from build123d import *

# Parameters (mm, degrees)
F0_R     = 21.614199
F1_DEPTH = 25.4


with BuildPart() as f1:
    # F0 (on Front) → F1 (new body)
    with BuildSketch(Plane.XZ):
        Polygon((-35.520531, 23.765538), (-35.520531, 0), (-35.520531, -26.832053), (-10.988366, -44.209), (-10.988366, -75.385295), (13.543796, -75.385295), (13.543796, -44.209), (38.075965, -26.832053), (38.075965, 0), (38.075965, 23.765538), align=None)
        Circle(F0_R, mode=Mode.SUBTRACT)
    extrude(amount=F1_DEPTH)


solid = f1.part
Here's how the part is built. I have some questions about the finished solid (model axes, mm). A direction names the side the tool comes from. Coordinates: 2 decimals unless noted, no trailing zeros. Order: outer loops, then holes, each group sorted by start corner. A loop starts at its lowest first (then second) coordinate and runs counter-clockwise, first axis right, second up.
Item 1: If we section it at A-A on y = -7.5: List the corners of the cut face in (x, z) for me.
Result sheet:
outline: (-35.52, -26.83) - (-10.99, -44.21) - (-10.99, -75.39) - (13.54, -75.39) - (13.54, -44.21) - (38.08, -26.83) - (38.08, 23.77) - (-35.52, 23.77) - close; hole circle Ø43.23 at (0, 0)
Item 2: I need wall thicknesses on line 1 (Z direction, x = 0, y = -13); line 2 (X direction, y = -22, z = -1); line 3 (X direction, y = -8.5, z = -56). Which ranges of each line are inside material? Lowest first, please.
Result sheet:
line 1: z = -75.39 to -21.61, 21.61 to 23.77
line 2: x = -35.52 to -21.59, 21.59 to 38.08
line 3: x = -10.99 to 13.54
Item 3: For faces 1 (the face through (13.544, -13, -60)), 2 (the face through (1, -13, -75.385)), which set-ups out of +Z, -Z, +X, -X, +Y, -Y let a thin tool reach every point of the face, with its end or its side?
Result sheet:
face 1: -Z, +X, +Y, -Y
face 2: -Z, +X, -X, +Y, -Y
Item 4: If we section it at D-D on x = 30.5: List the corners of the cut face in (y, z) for me.
Result sheet:
outline: (-25.4, -32.2) - (0, -32.2) - (0, 23.77) - (-25.4, 23.77) - close
Item 5: For P1, Ø2, axis at x = -14, y = -20.5, coming from the -Z side; P2, Ø1, axis at y = -6, z = -31.5, coming from the +X side; P3, Ø5, axis at x = -19.5, y = -5.5, coming from the -Z side, each with a flat end and sliding along its axis, tell me the tip position at first contact or that it passes through.
Result sheet:
P1: stops at z = -42.78
P2: stops at x = 32.19
P3: stops at z = -39.95
Item 6: If we section it at C-C on x = 0: List the corners of the cut face in (y, z) for me.
Result sheet:
outline: (-25.4, -75.39) - (0, -75.39) - (0, -21.61) - (-25.4, -21.61) - close; (-25.4, 21.61) - (0, 21.61) - (0, 23.77) - (-25.4, 23.77) - close
Item 7: If we section it at B-B on z = 0: List the corners of the cut face in (x, y) for me, plus the area to 3 significant figures.
Result sheet:
outline: (-35.52, -25.4) - (-21.61, -25.4) - (-21.61, 0) - (-35.52, 0) - close; (21.61, -25.4) - (38.08, -25.4) - (38.08, 0) - (21.61, 0) - close
area: 771 mm2
Item 8: If we mould it in two halves opening along X, with no side actions, what happens to faces 3 (the face through (-2.81, -12.52, 21.43)), 4 (the face through (-10.988, -13, -60)), 5 (the face through (25.64, -12.52, -35.64))? For each: +X half, -X half, draft (parallel to the pull), parting line (faces both ways), or undercut.
Result sheet:
face 3: undercut
face 4: -X half
face 5: +X half
